from build123d import *

# Parameters (mm, degrees)
SKETCH1_W           = 7.62
SKETCH1_H           = 30.48
SKETCH1_W_2         = 1.27
SKETCH1_H_2         = 1.27
BOSS_EXTRUDE1_DEPTH = 8.5852


with BuildPart() as part:
    # Sketch1 → Boss-Extrude1 (new body)
    with BuildSketch(Plane(origin=(0, 0, 0), x_dir=(1, 0, 0), z_dir=(0, 1, 0))):
        Rectangle(SKETCH1_W, SKETCH1_H)
        with Locations((-2.54, 13.97)):
            Rectangle(SKETCH1_W_2, SKETCH1_H_2, mode=Mode.SUBTRACT)
        with Locations((0, 13.97)):
            Rectangle(SKETCH1_W_2, SKETCH1_H_2, mode=Mode.SUBTRACT)
        with Locations((2.54, 13.97)):
            Rectangle(SKETCH1_W_2, SKETCH1_H_2, mode=Mode.SUBTRACT)
        with Locations((-2.54, 11.43)):
            Rectangle(SKETCH1_W_2, SKETCH1_H_2, mode=Mode.SUBTRACT)
        with Locations((0, 11.43)):
            Rectangle(SKETCH1_W_2, SKETCH1_H_2, mode=Mode.SUBTRACT)
        with Locations((2.54, 11.43)):
            Rectangle(SKETCH1_W_2, SKETCH1_H_2, mode=Mode.SUBTRACT)
        with Locations((-2.54, 8.89)):
            Rectangle(SKETCH1_W_2, SKETCH1_H_2, mode=Mode.SUBTRACT)
        with Locations((0, 8.89)):
            Rectangle(SKETCH1_W_2, SKETCH1_H_2, mode=Mode.SUBTRACT)
        with Locations((2.54, 8.89)):
            Rectangle(SKETCH1_W_2, SKETCH1_H_2, mode=Mode.SUBTRACT)
        with Locations((-2.54, 6.35)):
            Rectangle(SKETCH1_W_2, SKETCH1_H_2, mode=Mode.SUBTRACT)
        with Locations((0, 6.35)):
            Rectangle(SKETCH1_W_2, SKETCH1_H_2, mode=Mode.SUBTRACT)
        with Locations((2.54, 6.35)):
            Rectangle(SKETCH1_W_2, SKETCH1_H_2, mode=Mode.SUBTRACT)
        with Locations((-2.54, 3.81)):
            Rectangle(SKETCH1_W_2, SKETCH1_H_2, mode=Mode.SUBTRACT)
        with Locations((0, 3.81)):
            Rectangle(SKETCH1_W_2, SKETCH1_H_2, mode=Mode.SUBTRACT)
        with Locations((2.54, 3.81)):
            Rectangle(SKETCH1_W_2, SKETCH1_H_2, mode=Mode.SUBTRACT)
        with Locations((-2.54, 1.27)):
            Rectangle(SKETCH1_W_2, SKETCH1_H_2, mode=Mode.SUBTRACT)
        with Locations((0, 1.27)):
            Rectangle(SKETCH1_W_2, SKETCH1_H_2, mode=Mode.SUBTRACT)
        with Locations((2.54, 1.27)):
            Rectangle(SKETCH1_W_2, SKETCH1_H_2, mode=Mode.SUBTRACT)
        with Locations((-2.54, -1.27)):
            Rectangle(SKETCH1_W_2, SKETCH1_H_2, mode=Mode.SUBTRACT)
        with Locations((0, -1.27)):
            Rectangle(SKETCH1_W_2, SKETCH1_H_2, mode=Mode.SUBTRACT)
        with Locations((2.54, -1.27)):
            Rectangle(SKETCH1_W_2, SKETCH1_H_2, mode=Mode.SUBTRACT)
        with Locations((-2.54, -3.81)):
            Rectangle(SKETCH1_W_2, SKETCH1_H_2, mode=Mode.SUBTRACT)
        with Locations((0, -3.81)):
            Rectangle(SKETCH1_W_2, SKETCH1_H_2, mode=Mode.SUBTRACT)
        with Locations((2.54, -3.81)):
            Rectangle(SKETCH1_W_2, SKETCH1_H_2, mode=Mode.SUBTRACT)
        with Locations((-2.54, -6.35)):
            Rectangle(SKETCH1_W_2, SKETCH1_H_2, mode=Mode.SUBTRACT)
        with Locations((0, -6.35)):
            Rectangle(SKETCH1_W_2, SKETCH1_H_2, mode=Mode.SUBTRACT)
        with Locations((2.54, -6.35)):
            Rectangle(SKETCH1_W_2, SKETCH1_H_2, mode=Mode.SUBTRACT)
        with Locations((-2.54, -8.89)):
            Rectangle(SKETCH1_W_2, SKETCH1_H_2, mode=Mode.SUBTRACT)
        with Locations((0, -8.89)):
            Rectangle(SKETCH1_W_2, SKETCH1_H_2, mode=Mode.SUBTRACT)
        with Locations((2.54, -8.89)):
            Rectangle(SKETCH1_W_2, SKETCH1_H_2, mode=Mode.SUBTRACT)
        with Locations((-2.54, -11.43)):
            Rectangle(SKETCH1_W_2, SKETCH1_H_2, mode=Mode.SUBTRACT)
        with Locations((0, -11.43)):
            Rectangle(SKETCH1_W_2, SKETCH1_H_2, mode=Mode.SUBTRACT)
        with Locations((2.54, -11.43)):
            Rectangle(SKETCH1_W_2, SKETCH1_H_2, mode=Mode.SUBTRACT)
        with Locations((-2.54, -13.97)):
            Rectangle(SKETCH1_W_2, SKETCH1_H_2, mode=Mode.SUBTRACT)
        with Locations((0, -13.97)):
            Rectangle(SKETCH1_W_2, SKETCH1_H_2, mode=Mode.SUBTRACT)
        with Locations((2.54, -13.97)):
            Rectangle(SKETCH1_W_2, SKETCH1_H_2, mode=Mode.SUBTRACT)
    extrude(amount=BOSS_EXTRUDE1_DEPTH)


solid = part.part
Source: CAD feature listing. Evaluate the final solid. Frame: model axes, mm. Round coordinates to 2 decimals unless told otherwise and drop trailing zeros. Loops run counter-clockwise (first coordinate to the right, second up) from the corner with the lowest first, then second, coordinate; pieces in that order, holes last.
Q1. Ray query, line 1 (X direction, y = 4, z = 4) (3 decimals). Return the intervals inside material, ascending.
Q2. Mould query, pull axis Z, two halves, no side actions, for faces 1 (the face through (-3.175, 4, -14)), 2 (the face through (0, 4, -15.24)). Classes: pulls with the +Z half, pulls with the -Z half, needs draft (parallel to the pull), parting line crosses it, or undercut.
Q3. Section A-A, the plane z = -6.5. Return loops of the section in (x, y) (3 decimals).
Q4. Section B-B, the plane x = -2.5. State how many separate pieces and enclosed holes the cut face has, plus the area to 3 significant figures.
Solutions:
1. line 1: x = -3.81 to -3.175, -1.905 to -0.635, 0.635 to 1.905, 3.175 to 3.81
2. face 1: undercut
2. face 2: pulls with the -Z half
3. outline: (-3.81, 0) - (-3.175, 0) - (-3.175, 8.585) - (-3.81, 8.585) - close; (-1.905, 0) - (-0.635, 0) - (-0.635, 8.585) - (-1.905, 8.585) - close; (0.635, 0) - (1.905, 0) - (1.905, 8.585) - (0.635, 8.585) - close; (3.175, 0) - (3.81, 0) - (3.81, 8.585) - (3.175, 8.585) - close
4. separate pieces: 13
4. enclosed holes: 0
4. area: 131 mm2
